For this review, take the finished solid that the model builds, in its own axes (mm). A direction names the side the tool comes from. Give positions to 0.01 mm unless a question says otherwise; leave off trailing zeros. Loops run counter-clockwise (first coordinate to the right, second up) from the corner with the lowest first, then second, coordinate; pieces in that order, holes last.
Autodesk Inventor part; units mm, degrees
ref_plane "YZ Plane" through (0, 0, 0) normal (1, 0, 0) x (0, 1, 0)
ref_plane "XZ Plane" through (0, 0, 0) normal (0, 1, 0) x (-1, 0, 0)
ref_plane "XY Plane" through (0, 0, 0) normal (0, 0, 1) x (1, 0, 0)
sketch "Sketch1" plane through (0, 0, 0) normal (0, 0, 1) x (1, 0, 0)
  line L0 (-9, -3) -> (9, -3)
  line L1 (9, -3) -> (9, 3)
  line L2 (9, 3) -> (-9, 3)
  line L3 (-9, 3) -> (-9, -3)
  line L4 (-9, -3) -> (9, 3) construction
  line L5 (9, -3) -> (-9, 3) construction
  point P0 (0, 0)
  dimension "d0" = 18
  dimension "d1" = 6
extrude "Extrusion1" add sketch "Sketch1" along normal blind 3
sketch "Sketch2" plane through (0, 0, 3) normal (0, 0, 1) x (1, 0, 0)
  line L0 (-3, 3) -> (3, 3)
  line L1 (3, 3) -> (3, -3)
  line L2 (3, -3) -> (-3, -3)
  line L3 (-3, -3) -> (-3, 3)
  line L4 (-3, 3) -> (3, -3) construction
  line L5 (3, 3) -> (-3, -3) construction
  point P0 (0, 0)
  dimension "d4" = 6
  dimension "d5" = 6
extrude "Extrusion2" add sketch "Sketch2" along normal blind 40
sketch "Sketch3" plane through (0, 0, 43) normal (0, 0, 1) x (1, 0, 0)
  line L0 (9, 3) -> (-9, 3)
  line L1 (9, -3) -> (-9, -3)
  line L2 (-9, -3) -> (-9, 3)
  line L3 (-9, 3) -> (9, 3)
  line L4 (9, 3) -> (9, -3)
  line L5 (9, -3) -> (-9, 3) construction
  line L6 (-9, -3) -> (9, 3) construction
  point P0 (0, 0)
extrude "Extrusion3" add sketch "Sketch3" along normal blind 3
sketch "Sketch4" plane through (0, 0, 46) normal (0, 0, 1) x (1, 0, 0)
  circle A0 centre (6, 0) radius 1.5
  circle A1 centre (-6, 0) radius 1.5
  point P0 (0, 0)
  dimension "d10" = 3
  dimension "d11" = 3
extrude "Extrusion4" cut sketch "Sketch4" against normal up to surface (46 mm away)
properties part number "shaft"
Q1. For pin 1 Ø1.8 at (y, z) = (0, 31) entering from +X; pin 2 Ø3 at (y, z) = (0.5, 22.5) entering from -X; pin 3 Ø2.5 at (x, y) = (6, 0) entering from +Z, all flat-tipped, find the tip position at first contact; note any pin that passes through.
Answers:
pin 1: stops at x = 3
pin 2: stops at x = -3
pin 3: passes through
Q2. Consider section D-D on z = 7. Give the boundary of the cut face in (x, y), plus the area to 3 significant figures.
Answers:
outline: (-3, -3) - (3, -3) - (3, 3) - (-3, 3) - close
area: 36.0 mm2
Q3. For probe 1 along Z at (x, y) = (3.25, -1); probe 2 along Y at (x, z) = (6, 2.15); probe 3 along X at (y, z) = (2.8, 32), list the stretches that pass through material, from the lowest coordinate up.
Answers:
probe 1: z = 0 to 3, 43 to 46
probe 2: y = -3 to -1.5, 1.5 to 3
probe 3: x = -3 to 3
Q4. Consider section C-C on y = 2.2. Give the boundary of the cut face in (x, z), plus the area to 3 significant figures.
Answers:
outline: (-9, 0) - (9, 0) - (9, 3) - (3, 3) - (3, 43) - (9, 43) - (9, 46) - (-9, 46) - (-9, 43) - (-3, 43) - (-3, 3) - (-9, 3) - close
area: 348 mm2
Q5. Consider section A-A on y = 0. Give the boundary of the cut face in (x, z), plus the area to 3 significant figures.
Answers:
outline: (-9, 0) - (-7.5, 0) - (-7.5, 3) - (-9, 3) - close; (-9, 43) - (-7.5, 43) - (-7.5, 46) - (-9, 46) - close; (-4.5, 0) - (4.5, 0) - (4.5, 3) - (3, 3) - (3, 43) - (4.5, 43) - (4.5, 46) - (-4.5, 46) - (-4.5, 43) - (-3, 43) - (-3, 3) - (-4.5, 3) - close; (7.5, 0) - (9, 0) - (9, 3) - (7.5, 3) - close; (7.5, 43) - (9, 43) - (9, 46) - (7.5, 46) - close
area: 312 mm2
Q6. Machinability: for faces 5 (the flat face through (4.6, 1.4, 43)), 6 (the flat face through (-7.4, 1.4, 43)), 7 (the flat face through (9, 0, 44)), which of the approach directions +Z, -Z, +X, -X, +Y, -Y give a long, thin tool a straight path to every point of the face, cutting with its end or side? Answer none if there is none.
Answers:
face 5: +X, +Y, -Y
face 6: -X, +Y, -Y
face 7: +Z, -Z, +X, +Y, -Y
Q7. Mouldability with a two-part tool opening along Y and no side actions: class faces 1 (the cylindrical face through (-7.2, -0.9, 1.5)), 2 (the flat face through (0, -3, 23)), 3 (the flat face through (3, 0, 23)), 4 (the cylindrical face through (-7.2, -0.9, 44.5)) as +Y half, -Y half, draft (parallel to the pull), parting line (faces both ways), or undercut.
Answers:
face 1: undercut
face 2: -Y half
face 3: draft
face 4: undercut
Q8. Consider section B-B on x = -6. Give the boundary of the cut face in (y, z), plus the area to 3 significant figures.
Answers:
outline: (-3, 0) - (-1.5, 0) - (-1.5, 3) - (-3, 3) - close; (-3, 43) - (-1.5, 43) - (-1.5, 46) - (-3, 46) - close; (1.5, 0) - (3, 0) - (3, 3) - (1.5, 3) - close; (1.5, 43) - (3, 43) - (3, 46) - (1.5, 46) - close
area: 18.0 mm2
